Input: part model. Units: mm. Frame: model coordinates. A direction names the side the tool comes from. Coordinates: 2 decimals unless noted, no trailing zeros. Write each loop counter-clockwise with the first axis right and the second up, starting at its lowest first coordinate (ties: lowest second). Pieces come first, ordered by that corner, then holes.
1) Section query D-D (y = 4.95). Output: boundary loops of the cut face in (x, z).
2) Section query B-B (y = 0). Output: boundary loops of the cut face in (x, z).
3) Section query A-A (z = 24.3). Output: boundary loops of the cut face in (x, y), then the cut area to 3 significant figures.
4) Section query C-C (x = 6). Output: boundary loops of the cut face in (y, z), then the cut area to 3 significant figures.
5) Pin query (flat end, axial travel): pin 1 Ø5.5 at (x, z) = (14.5, 23.5) entering from -Y; pin 2 Ø5.5 at (y, z) = (0, 23.5) entering from -X; pin 3 Ø3 at (x, y) = (-18.5, 4.5) entering from +Z; pin 4 Ø3 at (y, z) = (4.95, -24.3) entering from +X. Return the tip coordinate at first contact, or that it passes through.
6) Set-up query: faces 1 (the flat face through (15, 0, 25)), 2 (the flat face through (-15, 0, 20)), 3 (the cylindrical face through (-8.6, -4.9, 21.8)), 4 (the flat face through (15, 3, 22)), 5 (the flat face through (12.25, 0, 22)). Return all of +Z, -Z, +X, -X, +Y, -Y with unobstructed straight access to the full face (end or side cutting, diameter ignored); none if empty.
7) Line query: L1, parallel to Y at x = -8.8, z = -24.3; L2, parallel to X at y = 7, z = -9.5; L3, parallel to Z at x = 8, y = 7.25. Output: solid intervals per line, ascending.
8) Draft query along Y for faces 6 (the cylindrical face through (-8.6, 4.9, -21.8)), 7 (the flat face through (7, 0, 20)), 8 (the flat face through (15, -3, 22)). Return one class per face: pulls with the +Y half, pulls with the -Y half, needs draft (parallel to the pull), parting line crosses it, or undercut.
from build123d import *

# Parameters (mm, degrees)
BOSS_EXTRUDE1_START = 20.25
SKETCH2_W           = 40
SKETCH2_H           = 20
SKETCH2_R           = 3
BOSS_EXTRUDE1_DEPTH = 40.5
BOSS_EXTRUDE2_START = -7.05
BOSS_EXTRUDE2_DEPTH = 3.2
BOSS_EXTRUDE3_START = -20.25
SKETCH2_5_R         = 3
BOSS_EXTRUDE3_DEPTH = 5.5
SKETCH3_W           = 5
SKETCH3_H           = 6
BOSS_EXTRUDE4_DEPTH = 5


with BuildPart() as part:
    # Sketch2 → Boss-Extrude1 (new body)
    # profile 1 of 2: a face of its own
    with BuildSketch(Plane(origin=(0, 0, 0), x_dir=(0, 0, -1), z_dir=(1, 0, 0)).offset(BOSS_EXTRUDE1_START)):
        Rectangle(SKETCH2_W, SKETCH2_H)
        with Locations((-10.2, 0)):
            Circle(SKETCH2_R, mode=Mode.SUBTRACT)
    # profile 2 of 2: a face of its own
    with BuildSketch(Plane(origin=(0, 0, 0), x_dir=(0, 0, -1), z_dir=(1, 0, 0)).offset(BOSS_EXTRUDE1_START)):
        with Locations((-10.2, 0)):
            Circle(SKETCH2_R)
    extrude(amount=-BOSS_EXTRUDE1_DEPTH)

    # Sketch2<3> → Boss-Extrude2 (add)
    with BuildSketch(Plane(origin=(0, 0, 0), x_dir=(0, 0, -1), z_dir=(1, 0, 0)).offset(BOSS_EXTRUDE2_START)):
        with BuildLine():
            Line((-26, -10), (-20, -10))
            Line((-20, -10), (-20, 10))
            Line((-20, 10), (-26, 10))
            Line((-26, 10), (-26, 6.783030278))
            ThreePointArc((-26, 6.783030278), (-21.8, 4.95), (-26, 3.116969722))
            Line((-26, 3.116969722), (-26, -3.116969722))
            ThreePointArc((-26, -3.116969722), (-21.8, -4.95), (-26, -6.783030278))
            Line((-26, -6.783030278), (-26, -10))
        make_face()
        with BuildLine():
            Line((20, 10), (20, -10))
            Line((20, -10), (26, -10))
            Line((26, -10), (26, -6.783030278))
            ThreePointArc((26, -6.783030278), (21.8, -4.95), (26, -3.116969722))
            Line((26, -3.116969722), (26, 3.116969722))
            ThreePointArc((26, 3.116969722), (21.8, 4.95), (26, 6.783030278))
            Line((26, 6.783030278), (26, 10))
            Line((26, 10), (20, 10))
        make_face()
    extrude(amount=-BOSS_EXTRUDE2_DEPTH)

    # Sketch2<5> → Boss-Extrude3 (add)
    with BuildSketch(Plane(origin=(0, 0, 0), x_dir=(0, 0, -1), z_dir=(1, 0, 0)).offset(BOSS_EXTRUDE3_START)):
        with Locations((-10.2, 0)):
            Circle(SKETCH2_5_R)
    extrude(amount=-BOSS_EXTRUDE3_DEPTH)

    # Sketch3 → Boss-Extrude4 (add)
    with BuildSketch(Plane.XY.offset(20)):
        with Locations((14.75, 0)):
            Rectangle(SKETCH3_W, SKETCH3_H)
    extrude(amount=BOSS_EXTRUDE4_DEPTH)


solid = part.part
Answer:
1. outline: (-20.25, -20) - (-10.25, -20) - (-10.25, -21.8) - (-7.05, -21.8) - (-7.05, -20) - (20.25, -20) - (20.25, 20) - (-7.05, 20) - (-7.05, 21.8) - (-10.25, 21.8) - (-10.25, 20) - (-20.25, 20) - close
2. outline: (-25.75, 7.2) - (-20.25, 7.2) - (-20.25, -20) - (-10.25, -20) - (-10.25, -26) - (-7.05, -26) - (-7.05, -20) - (20.25, -20) - (20.25, 20) - (17.25, 20) - (17.25, 25) - (12.25, 25) - (12.25, 20) - (-7.05, 20) - (-7.05, 26) - (-10.25, 26) - (-10.25, 20) - (-20.25, 20) - (-20.25, 13.2) - (-25.75, 13.2) - close
3. outline: (-10.25, -10) - (-7.05, -10) - (-7.05, -7.45) - (-10.25, -7.45) - close; (-10.25, -2.45) - (-7.05, -2.45) - (-7.05, 2.45) - (-10.25, 2.45) - close; (-10.25, 7.45) - (-7.05, 7.45) - (-7.05, 10) - (-10.25, 10) - close; (12.25, -3) - (17.25, -3) - (17.25, 3) - (12.25, 3) - close
3. area: 62.0 mm2
4. outline: (-10, -20) - (10, -20) - (10, 20) - (-10, 20) - close
4. area: 800 mm2
5. pin 1: stops at y = -3
5. pin 2: stops at x = -10.25
5. pin 3: stops at z = 20
5. pin 4: passes through
6. face 1: +Z, +X, +Y, -Y
6. face 2: +Z, -X, +Y, -Y
6. face 3: -X
6. face 4: +Z, +X, +Y
6. face 5: +Z, +Y, -Y
7. L1: y = -10 to -7.45, -2.45 to 2.45, 7.45 to 10
7. L2: x = -20.25 to 20.25
7. L3: z = -20 to 20
8. face 6: undercut
8. face 7: needs draft
8. face 8: pulls with the -Y half
